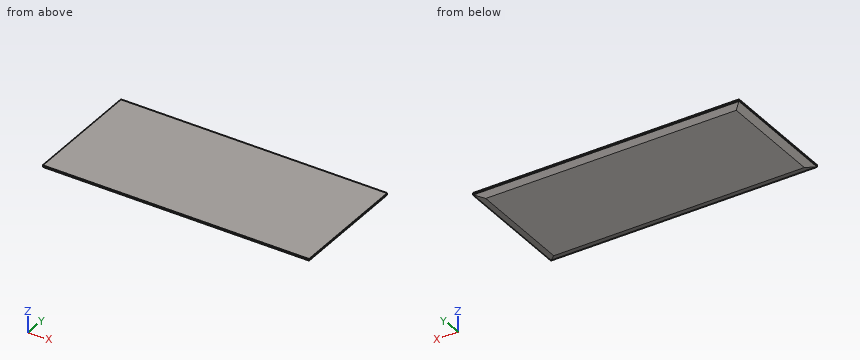
from build123d import *

# Parameters (mm, degrees)
F0_W     = 1676.4
F0_H     = 762
F1_DEPTH = 24
F5_R     = 5


with BuildPart() as f1:
    # F0 (on Top) → F1 (new body)
    with BuildSketch(Plane.XY):
        Rectangle(F0_W, F0_H)
    extrude(amount=F1_DEPTH)

    # F4: sweep along a path in F3
    with BuildLine(Plane(origin=(0, 0, 0), x_dir=(1, 0, 0), z_dir=(0, 0, -1))) as f4_path:
        Line((838.2, 381), (-838.2, 381))
        Line((-838.2, 381), (-838.2, -381))
        Line((-838.2, -381), (838.2, -381))
        Line((838.2, -381), (838.2, 381))
    # F2 (on face) → F4 (sweep, cut)
    with BuildSketch(Plane.YZ.offset(838.2)):
        Polygon((381, 14), (331, 0), (381, 0), align=None)
    sweep(path=f4_path.line, transition=Transition.RIGHT, mode=Mode.SUBTRACT)

    # F5
    f5_edges = [f1.edges().sort_by_distance(p)[0] for p in [
        (838.2, 381, 19),
        (838.2, -381, 19),
        (-838.2, 381, 19),
        (-838.2, -381, 19),
    ]]
    fillet(f5_edges, radius=F5_R)


solid = f1.part
Here's how the part is built. I have some questions about the finished solid (model axes, mm). Give positions to 0.01 mm unless a question says otherwise; leave off trailing zeros. Loops run counter-clockwise (first coordinate to the right, second up) from the corner with the lowest first, then second, coordinate; pieces in that order, holes last. Notation, with made-up numbers: (74.25, -8.75) -> (98.25, -8.75) arc R20 cw to (98.25, 19.25) -> close; hole circle Ø2 at (73.25, 22.25). An arc over 180 degrees is marked (long way). Answer as a JSON object with one key per item and string values. Group by question number.
Item 1: Imagine slicing it at A-A on y = 178. Write out the boundary of the cut face in (x, z), then the cut area to 3 significant figures.
Item 2: Imagine slicing it at B-B on x = 696. Write out the boundary of the cut face in (y, z), then the cut area to 3 significant figures.
Item 3: I need wall thicknesses on L1, parallel to Z at x = 687.5, y = -335; L2, parallel to Z at x = -421, y = 338. Which ranges of each line are inside material? Lowest first, please.
Item 4: Imagine slicing it at C-C on z = 7. Write out the boundary of the cut face in (x, y), then the cut area to 3 significant figures.
Answer list:
{
 "1": {"outline": "(-838.2, 14) -> (-788.2, 0) -> (788.2, 0) -> (838.2, 14) -> (838.2, 24) -> (-838.2, 24) -> close", "area": "39,500 mm2"},
 "2": {"outline": "(-381, 14) -> (-331, 0) -> (331, 0) -> (381, 14) -> (381, 24) -> (-381, 24) -> close", "area": "17,600 mm2"},
 "3": {"L1": "z = 1.12 to 24", "L2": "z = 1.96 to 24"},
 "4": {"outline": "(-813.2, -356) -> (813.2, -356) -> (813.2, 356) -> (-813.2, 356) -> close", "area": "1,160,000 mm2"}
}
